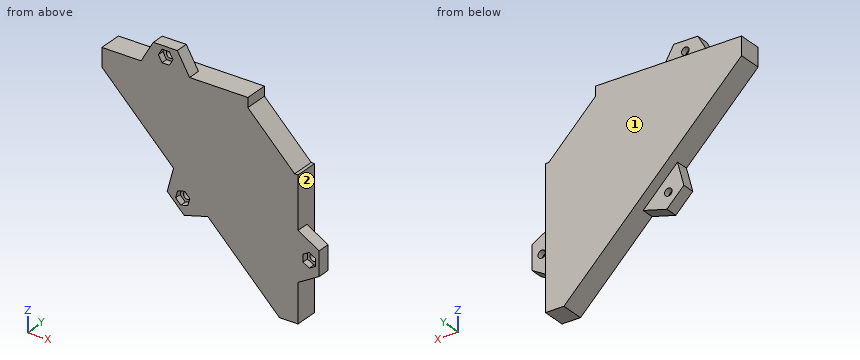
```python
from build123d import *

# Parameters (mm, degrees)
BOSS_EXTRUDE1_DEPTH = 13
BOSS_EXTRUDE2_DEPTH = 7
SKETCH3_R           = 2.1
CUT_EXTRUDE1_DEPTH  = 293.087257838
CUT_EXTRUDE2_DEPTH  = 3.5


with BuildPart() as part:
    # Sketch1 → Boss-Extrude1 (new body)
    with BuildSketch(Plane(origin=(0, -14.270631866, 0), x_dir=(-1, 0, 0), z_dir=(0, -1, 0))):
        Polygon((-95.804533303, -147.092026732), (2.510114699, -245.053270909), (2.510114699, -255.216605782), (-78.283971389, -255.216605782), (-78.283971389, -249.988254121), (-104.187777311, -224.084448198), (-106.041330702, -224.084448198), (-106.041330702, -147.092026732), align=None)
    extrude(amount=-BOSS_EXTRUDE1_DEPTH)

    # Sketch2 → Boss-Extrude2 (add)
    with BuildSketch(Plane.XZ.offset(14.270631866)):
        Polygon((37.243094616, 205.795877803), (-2.510114699, 245.406189427), (-2.510114699, 254.966605782), (19.041650219, 254.966605782), (25.96985345, 266.966605782), (39.248909641, 266.966605782), (46.177112871, 254.966605782), (78.033971389, 254.966605782), (78.033971389, 249.88470073), (104.084223921, 223.834448198), (105.791330702, 223.834448198), (105.791330702, 195.567357996), (117.791330702, 188.639154765), (117.791330702, 175.360098574), (105.791330702, 168.431895344), (105.791330702, 147.092026732), (96.158725005, 147.092026732), (56.444502381, 186.663491807), (43.053372765, 183.04954817), (33.664085816, 192.438835119), align=None)
    extrude(amount=-BOSS_EXTRUDE2_DEPTH)

    # Sketch3 → Cut-Extrude1 (cut, through all)
    with BuildSketch(Plane.XZ.offset(14.270631866)):
        with Locations(Location((42.248028453, 191.633067075, 0), (0, 0, 270))):
            Circle(SKETCH3_R)
        with Locations(Location((32.824351589, 261.466605782, 0), (0, 0, 270))):
            Circle(SKETCH3_R)
        with Locations(Location((112.291330702, 181.99962667, 0), (0, 0, 270))):
            Circle(SKETCH3_R)
    extrude(amount=-CUT_EXTRUDE1_DEPTH, mode=Mode.SUBTRACT)

    # Sketch4 → Cut-Extrude2 (cut)
    with BuildSketch(Plane.XZ.offset(14.270631866)):
        Polygon((36.865803473, 261.466605782), (34.845077531, 264.966605782), (30.803625647, 264.966605782), (28.782899705, 261.466605782), (30.803625647, 257.966605782), (34.845077531, 257.966605782), align=None)
        Polygon((46.151771204, 192.679071793), (43.29403317, 195.536809826), (39.39029042, 194.490805109), (38.344285702, 190.587062358), (41.202023735, 187.729324324), (45.105766486, 188.775329042), align=None)
        Polygon((108.791330702, 184.020352612), (108.791330702, 179.978900727), (112.291330702, 177.958174785), (115.791330702, 179.978900727), (115.791330702, 184.020352612), (112.291330702, 186.041078554), align=None)
    extrude(amount=-CUT_EXTRUDE2_DEPTH, mode=Mode.SUBTRACT)


solid = part.part
```
Verification items for the finished model (mm, model axes). Face numbers are marked on the shaded views. A direction names the side the tool comes from. Give positions to 0.01 mm unless a question says otherwise; leave off trailing zeros. Order: outer loops, then holes, each group sorted by start corner. A loop starts at its lowest first (then second) coordinate and runs counter-clockwise, first axis right, second up. Notation, with made-up numbers: (-35, -8) -> (-6, -8) arc R30 cw to (-6, 27) -> close; hole circle Ø9 at (46, -14.5). An arc over 180 degrees is marked (long way). Use a Markdown table: item, result.
1) Tool access check on the marked faces 1 and 2. Record the directions out of +Z, -Z, +X, -X, +Y, -Y that give a thin tool (end or side, any length) a straight path to the whole face; none if there is none.
Results:
| item | result |
|---|---|
| face 1 | +Z, -Z, +X, -X, +Y |
| face 2 | +X, +Y |
2) Section check B-B, the plane z = 198.5. Record the boundary of the cut face in (x, y), then the cut area to 3 significant figures.
Results:
| item | result |
|---|---|
| outline | (35.29, -14.27) -> (106.04, -14.27) -> (106.04, -1.27) -> (44.21, -1.27) -> (44.21, -7.27) -> (35.29, -7.27) -> close |
| area | 866 mm² |
3) Section check D-D, the plane x = 74. Record the boundary of the cut face in (y, z).
Results:
| item | result |
|---|---|
| outline | (-14.27, 168.82) -> (-1.27, 168.82) -> (-1.27, 255.22) -> (-14.27, 255.22) -> close |
4) Section check A-A, the plane y = -3. Record the boundary of the cut face in (x, z).
Results:
| item | result |
|---|---|
| outline | (-2.51, 245.05) -> (95.8, 147.09) -> (106.04, 147.09) -> (106.04, 224.08) -> (104.19, 224.08) -> (78.28, 249.99) -> (78.28, 255.22) -> (-2.51, 255.22) -> close |
5) Material ranges on probe 1 along X at (y, z) = (-6, 250); probe 2 along Y at (x, z) = (49.5, 185); probe 3 along Z at (x, y) = (105, -5), recorded low to high.
Results:
| item | result |
|---|---|
| probe 1 | -2.51 to 78.28 |
| probe 2 | -14.27 to -7.27 |
| probe 3 | 147.09 to 224.08 |
6) Depth check by flat-ended pin: pin 1 Ø2 at (x, y) = (56, -12.5) entering from +Z; pin 2 Ø3 at (y, z) = (-12.5, 182.5) entering from -X; pin 3 Ø6.5 at (x, z) = (43, 193) entering from +Y; pin 4 Ø4 at (x, z) = (42.25, 191.63) entering from +Y. Enter the tip coordinate at first touch or a pass-through.
Results:
| item | result |
|---|---|
| pin 1 | z = 255.22 |
| pin 2 | x = 42.1 |
| pin 3 | y = -7.27 |
| pin 4 | through |
7) Section check C-C, the plane y = -12.25. Give the number of separate pieces and of enclosed holes in the cut face, then the cut area to 3 significant figures.
Results:
| item | result |
|---|---|
| separate pieces | 1 |
| enclosed holes | 3 |
| area | 6,970 mm² |
